Part model, mm, in its own coordinate system. Face numbers are marked on the shaded views. A direction names the side the tool comes from. Round coordinates to 2 decimals unless told otherwise and drop trailing zeros. Order: outer loops, then holes, each group sorted by start corner. A loop starts at its lowest first (then second) coordinate and runs counter-clockwise, first axis right, second up. Notation, with made-up numbers: (20.25, 82) - (40.25, 82) arc R21 cw to (40.25, 116) - close; hole circle Ø10 at (52.25, -0.75). An arc over 180 degrees is marked (long way). Return JSON: item names as keys, results as strings. Group by question number.
Item 1: Saw through at B-B on z = 9.5. List the corners of the cut face in (x, y), and give its area (3 significant figures).
Item 2: Tool access for the marked faces 1, 2 and 3: list every direction of +Z, -Z, +X, -X, +Y, -Y with a clear straight run to the whole face (end or side of a thin tool).
Item 3: Probe probe 1 along X at (y, z) = (2.1, 9.5); probe 2 along Y at (x, z) = (7, -0.5); probe 3 along Z at (x, y) = (9.5, 4). List the from-to ranges inside material, lowest first.
Item 4: Saw through at C-C on y = 24.5. List the corners of the cut face in (x, z), and give its area (3 significant figures).
Item 5: Drop flat-ended pins along their axis: pin 1 (2.5 mm diameter, centred on x = 10, z = 9.5, fed in from +Y); pin 2 (6 mm diameter, centred on y = 14, z = -1, fed in from +X); pin 3 (9.5 mm diameter, centred on x = -1, z = 7, fed in from +Y); pin 4 (6 mm diameter, centred on x = -4, y = 29.5, fed in from +Z). Give the stop position or say it passes through.
Item 6: Saw through at A-A on x = 10. List the corners of the cut face in (y, z).
Item 7: Saw through at D-D on x = 3.5. List the corners of the cut face in (y, z).
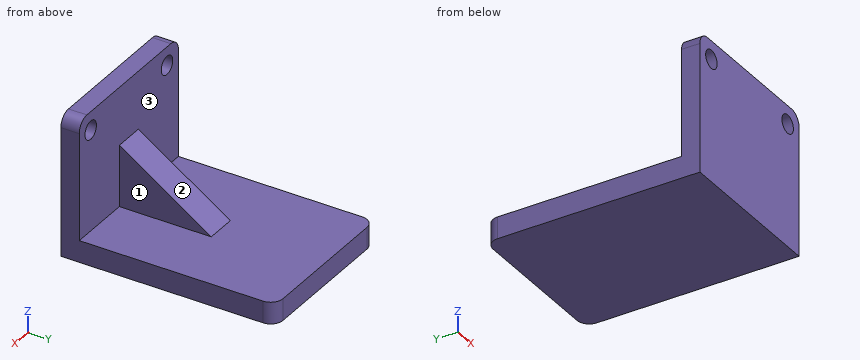
```python
from build123d import *

# Parameters (mm, degrees)
SKETCH1_R           = 1.5
BOSS_EXTRUDE1_DEPTH = 3
SKETCH2_W           = 3.546458452
SKETCH2_H           = 32
BOSS_EXTRUDE2_DEPTH = 26
BOSS_EXTRUDE3_START = -10.5
BOSS_EXTRUDE3_DEPTH = 5
FILLET1_R           = 2
FILLET2_R           = 2


with BuildPart() as part:
    # Sketch1 → Boss-Extrude1 (new body)
    with BuildSketch(Plane(origin=(0, 0, 0), x_dir=(1, 0, 0), z_dir=(0, 1, 0))):
        with BuildLine():
            Line((13, 10.5), (-13, 10.5))
            Line((-13, 10.5), (-13, -10.5))
            ThreePointArc((-13, -10.5), (-12.414213562, -11.914213562), (-11, -12.5))
            Line((-11, -12.5), (11, -12.5))
            ThreePointArc((11, -12.5), (12.414213562, -11.914213562), (13, -10.5))
            Line((13, -10.5), (13, 10.5))
        make_face()
        with Locations(Location((-10, -9.5, 0), (0, 0, 270))):
            Circle(SKETCH1_R, mode=Mode.SUBTRACT)
        with Locations(Location((10, -9.5, 0), (0, 0, 270))):
            Circle(SKETCH1_R, mode=Mode.SUBTRACT)
    extrude(amount=BOSS_EXTRUDE1_DEPTH)

    # Sketch2 → Boss-Extrude2 (add)
    with BuildSketch(Plane.ZY.offset(13)):
        with Locations((-8.726770774, 19)):
            Rectangle(SKETCH2_W, SKETCH2_H)
    extrude(amount=-BOSS_EXTRUDE2_DEPTH)

    # Sketch3 → Boss-Extrude3 (add)
    with BuildSketch(Plane.ZY.offset(13).offset(BOSS_EXTRUDE3_START)):
        Polygon((-6.953541548, 18), (3.046458452, 3), (-6.953541548, 3), align=None)
    extrude(amount=-BOSS_EXTRUDE3_DEPTH)

    # Fillet1
    fillet1_edges = [part.edges().sort_by_distance(p)[0] for p in [
        (-13, 35, -8.726770774),
    ]]
    fillet(fillet1_edges, radius=FILLET1_R)

    # Fillet2
    fillet2_edges = [part.edges().sort_by_distance(p)[0] for p in [
        (13, 35, -8.726770774),
    ]]
    fillet(fillet2_edges, radius=FILLET2_R)


solid = part.part
```
Filled in:
{
 "1": {"outline": "(-13, 0) - (-11.5, 0) - (-11.5, 3) - (-13, 3) - close; (-8.5, 0) - (8.5, 0) - (8.5, 3) - (-8.5, 3) - close; (11.5, 0) - (13, 0) - (13, 3) - (11.5, 3) - close", "area": "60.0 mm^2"},
 "2": {"face 1": "+Z, +X, +Y", "face 2": "+Z, +X, -X, +Y", "face 3": "+Z, +Y"},
 "3": {"probe 1": "x = -13 to -11.5, -8.5 to 8.5, 11.5 to 13", "probe 2": "y = 0 to 3", "probe 3": "z = -10.5 to -6.95"},
 "4": {"outline": "(-13, -10.5) - (13, -10.5) - (13, -6.95) - (-13, -6.95) - close", "area": "92.2 mm^2"},
 "5": {"pin 1": "passes through", "pin 2": "stops at x = 2.5", "pin 3": "stops at y = 4.19", "pin 4": "stops at z = -6.95"},
 "6": {"outline": "(0, -10.5) - (35, -10.5) - (35, -6.95) - (3, -6.95) - (3, 8) - (0, 8) - close; (0, 11) - (3, 11) - (3, 12.5) - (0, 12.5) - close"},
 "7": {"outline": "(0, -10.5) - (35, -10.5) - (35, -6.95) - (3, -6.95) - (3, 12.5) - (0, 12.5) - close"}
}
